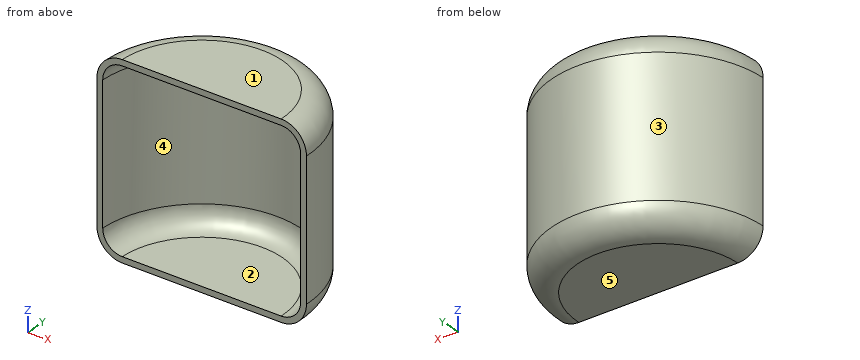
```python
from build123d import *

# Parameters (mm, degrees)
F1_DEPTH = 406.4
F2_R     = 55.1942
F4_T     = -12.7


# Not quite as in the source:
# - two fillets or chamfers of one size are made in one step


with BuildPart() as f1:
    # F0 (on Top) → F1 (new body)
    with BuildSketch(Plane.XY):
        with BuildLine():
            ThreePointArc((228.6, 0), (0, 228.6), (-228.6, 0))
            Line((-228.6, 0), (228.6, 0))
        make_face()
    extrude(amount=F1_DEPTH)

    # F2
    f2_edges = [f1.edges().sort_by_distance(p)[0] for p in [
        (0, 228.6, 406.4),
        (0, 228.6, 0),
    ]]
    fillet(f2_edges, radius=F2_R)

    # F4
    f4_openings = [f1.faces().sort_by_distance(p)[0] for p in [
        (0, 0, 203.2),
    ]]
    offset(amount=F4_T, openings=f4_openings)


solid = f1.part
```
Input: part model. Units: mm. Frame: model coordinates. Face numbers are marked on the shaded views. A direction names the side the tool comes from. Give positions to 0.01 mm unless a question says otherwise; leave off trailing zeros. Order: outer loops, then holes, each group sorted by start corner. A loop starts at its lowest first (then second) coordinate and runs counter-clockwise, first axis right, second up. Notation, with made-up numbers: M 58.25,50.5 L 88.25,50.5 A18 ccw 88.25,57.5 Z; hole C -16,1 d4. An arc over 180 degrees is marked long. One line per question, with ' | ' between items. Start each with the question number.
1. Material intervals for probe 1 along Z at (x, y) = (14.5, 49.5); probe 2 along X at (y, z) = (178.5, 241.5); probe 3 along X at (y, z) = (50, 350.5), sorted ascending. Write a range as [from, to].
2. Section query B-B (z = 105). Return the cut outline in (x, y).
3. First-contact query: pin 1 Ø5 at (y, z) = (71, 361.5) entering from -X; pin 2 Ø6 at (y, z) = (175.5, 60) entering from +X; pin 3 Ø10 at (x, z) = (131.5, 363) entering from -Y. Flat tips, straight axial feed; report the tip coordinate or a pass-through.
4. Section query A-A (x = 0). Return the cut outline in (y, z).
5. Access query for the marked faces 1 and 2. Directions: +Z, -Z, +X, -X, +Y, -Y. A direction counts if a zero-diameter tool reaches every point of the face in a straight line with its end or side. Return the directions, or none.
6. Pull-direction query (X, two-part tool) for the marked faces 3, 4 and 5; classes: released by +X, released by -X, zero draft, split by the parting line, or undercut.
Here are the results:
1) probe 1: [0, 12.7], [393.7, 406.4] | probe 2: [-142.81, -121.45], [121.45, 142.81] | probe 3: [-223.06, -210.03], [210.03, 223.06]
2) outline: M -228.6,0 L -215.9,0 A215.9 cw 215.9,0 L 228.6,0 A228.6 ccw Z
3) pin 1: x = -217.21 | pin 2: x = 150.01 | pin 3: y = 164.62
4) outline: M 0,0 L 173.41,0 A55.19 ccw 228.6,55.19 L 228.6,351.21 A55.19 ccw 173.41,406.4 L 0,406.4 L 0,393.7 L 173.41,393.7 A42.49 cw 215.9,351.21 L 215.9,55.19 A42.49 cw 173.41,12.7 L 0,12.7 Z
5) face 1: +Z, +X, -X, +Y, -Y | face 2: -Y
6) face 3: split by the parting line | face 4: undercut | face 5: zero draft
